Part model, mm, in its own coordinate system. Coordinates: 2 decimals unless noted, no trailing zeros. Loops run counter-clockwise (first coordinate to the right, second up) from the corner with the lowest first, then second, coordinate; pieces in that order, holes last. Notation, with made-up numbers: (-32, 75.5) - (-5, 75.5) arc R25 ccw to (-5, 114.5) - close; hole circle Ø9 at (15.25, 61.25). An arc over 180 degrees is marked (long way). Answer as CSV lines item,"result".
from build123d import *

# Parameters (mm, degrees)
F0_R     = 25
F1_DEPTH = 20


with BuildPart() as f1:
    # F0 (on Front) → F1 (new body)
    with BuildSketch(Plane.XZ):
        with BuildLine():
            ThreePointArc((47.017566, 205.35291), (49.248748, 196.977526), (50, 188.342663))
            ThreePointArc((50, 188.342663), (-8.634863, 139.093915), (-47.017566, 205.35291))
            Line((-47.017566, 205.35291), (-140, -51.657337))
            Line((-140, -51.657337), (140, -51.657337))
            Line((140, -51.657337), (47.017566, 205.35291))
        make_face()
        with BuildLine():
            ThreePointArc((-47.017566, 205.35291), (-8.634863, 139.093915), (50, 188.342663))
            ThreePointArc((50, 188.342663), (49.248748, 196.977526), (47.017566, 205.35291))
            ThreePointArc((47.017566, 205.35291), (0, 238.342663), (-47.017566, 205.35291))
        make_face()
        with Locations((0, 188.342663)):
            Circle(F0_R, mode=Mode.SUBTRACT)
    extrude(amount=F1_DEPTH)


solid = f1.part
Q1. Saw through at B-B (z = 210). Give the cut face in (x, y).
Results:
outline,"(-45.07, -20) - (-12.49, -20) - (-12.49, 0) - (-45.07, 0) - close; (12.49, -20) - (45.07, -20) - (45.07, 0) - (12.49, 0) - close"
Q2. Two-plate mould, pull along Z, no slides. Class faces 1 (the face through (94.16, -9.86, 75.05)), 2 (the face through (-3.25, -9.86, 213.13)), 3 (the face through (-2, -10, -51.657)): released by +Z, released by -Z, zero draft, split by the parting line, or undercut.
Results:
face 1,"released by +Z"
face 2,"undercut"
face 3,"released by -Z"
Q3. Wall check: L1, parallel to X at y = -1.25, z = 195; L2, parallel to Z at x = -4.5, y = -8.75; L3, parallel to X at y = -9, z = 191.5. Give the ranges that are in metal, low to high.
Results:
L1,"x = -50.76 to -24.1, 24.1 to 50.76"
L2,"z = -51.66 to 163.75, 212.93 to 238.14"
L3,"x = -52.03 to -24.8, 24.8 to 52.03"
Q4. Flat gauge pins, fed straight in: pin 1 (6 mm diameter, centred on x = 38, y = -6, fed in from +Z); pin 2 (1 mm diameter, centred on y = -13.5, z = 62, fed in from +X); pin 3 (2 mm diameter, centred on y = -3.5, z = 175, fed in from -X). Where does each tip first touch, or does it go through?
Results:
pin 1,"stops at z = 224.05"
pin 2,"stops at x = 99.06"
pin 3,"stops at x = -58.36"
Q5. Saw through at C-C (y = -15). Give the cut face in (x, z), then the cut area to 3 significant figures.
Results:
outline,"(-140, -51.66) - (140, -51.66) - (47.02, 205.35) arc R50 ccw to (-47.02, 205.35) - close; hole circle Ø50 at (0, 188.34)"
area,"48,400 mm^2"
Q6. Saw through at A-A (x = 0). Give the cut face in (y, z), then the cut area to 3 significant figures.
Results:
outline,"(-20, -51.66) - (0, -51.66) - (0, 163.34) - (-20, 163.34) - close; (-20, 213.34) - (0, 213.34) - (0, 238.34) - (-20, 238.34) - close"
area,"4,800 mm^2"
Q7. Saw through at D-D (z = -20). Give the cut face in (x, y), then the cut area to 3 significant figures.
Results:
outline,"(-128.55, -20) - (128.55, -20) - (128.55, 0) - (-128.55, 0) - close"
area,"5,140 mm^2"
